Check sheet for the modelled part. Datum: model origin and axes. Units: mm. A direction names the side the tool comes from. Coordinates: 2 decimals unless noted, no trailing zeros. Loops run counter-clockwise (first coordinate to the right, second up) from the corner with the lowest first, then second, coordinate; pieces in that order, holes last. Notation, with made-up numbers: (51.5, 77) - (79.5, 77) arc R21 ccw to (79.5, 111) - close; hole circle Ø4 at (-29.75, 41.25). An arc over 180 degrees is marked (long way). Use a Markdown table: item, result. Add a question column.
1) Sectioned sample at A-A, the plane y = 6. Enter the section's corners in (x, z).
2) Go/stop test with flat-tipped pins: P1, Ø1.5, axis at x = 6, y = 3, coming from the +Z side; P2, Ø3.5, axis at y = 6, z = 0, coming from the -X side; P3, Ø3, axis at x = 4.5, y = 1, coming from the -Z side; P4, Ø2, axis at x = -1, z = -1.5, coming from the +Y side. Record where each tip stops, or that it passes through.
3) Draft check along Z on faces 4 (the cylindrical face through (-1.216, 0.021, 1.115)), 5 (the cylindrical face through (6.47, 8.93, 1.84)), 6 (the flat face through (5.4, 1.9, -2.6)). Enter one of: pulls with the +Z half, pulls with the -Z half, needs draft (parallel to the pull), parting line crosses it, or undercut.
4) Tool access check on faces 1 (the flat face through (7.741, 3, 0)), 2 (the flat face through (5.4, 1.9, 2.443)), 3 (the flat face through (2, 1.5, 0)). Record the directions out of +Z, -Z, +X, -X, +Y, -Y that give a thin tool (end or side, any length) a straight path to the whole face; none if there is none.
5) Sectioned sample at D-D, the plane x = 4. Enter the section's corners in (y, z).
6) Sectioned sample at C-C, the plane z = 0. Enter the section's corners in (x, y), then the cut area to 3 significant figures.
7) Sectioned sample at B-B, the plane x = 0. Enter the section's corners in (y, z).
8) Thickness scan on line 1 (Z direction, x = 6, y = 6); line 2 (Z direction, x = 0, y = 0.8); line 3 (X direction, y = 1.75, z = 0.45). Record the ranges inside material, lowest first.
from build123d import *

# Parameters (mm, degrees)
F0_R          = 3
F0_R_2        = 1.65
F1_DEPTH      = 1.5
F1_DEPTH_BACK = 1.5
F3_DEPTH      = 1.5
F3_DEPTH_BACK = 1.5
F4_W          = 2.5
F4_H          = 5.04355
F5_DEPTH      = 8
F6_R          = 2.05
F7_DEPTH      = 25
F8_R          = 2


with BuildPart() as f1:
    # F0 (on Front) → F1 (new body, two sides)
    with BuildSketch(Plane.XZ) as f1_sk:
        Circle(F0_R)
        Circle(F0_R_2, mode=Mode.SUBTRACT)
    extrude(amount=F1_DEPTH)
    extrude(f1_sk.sketch, amount=-F1_DEPTH_BACK)

    # F2 (on Front) → F3 (join, two sides)
    with BuildSketch(Plane.XZ) as f3_sk:
        with BuildLine():
            Line((7.740623, 2.443406), (1.740623, 2.443406))
            ThreePointArc((1.740623, 2.443406), (2.666633, 1.374433), (3, 0))
            ThreePointArc((3, 0), (2.59704, -1.501793), (1.496413, -2.600144))
            Line((1.496413, -2.600144), (7.740623, -2.600144))
            Line((7.740623, -2.600144), (7.740623, 2.443406))
        make_face()
    extrude(amount=F3_DEPTH)
    extrude(f3_sk.sketch, amount=-F3_DEPTH_BACK)

    # F4 (on face) → F5 (join)
    with BuildSketch(Plane(origin=(0, 1.5, 0), x_dir=(-1, 0, 0), z_dir=(0, 1, 0))):
        with Locations((-6.490623, -0.078369)):
            Rectangle(F4_W, F4_H)
    extrude(amount=F5_DEPTH)

    # F6 (on face) → F7 (cut)
    with BuildSketch(Plane(origin=(5.240623, 0, 0), x_dir=(0, -1, 0), z_dir=(-1, 0, 0))):
        with Locations((-6, 0)):
            Circle(F6_R)
    extrude(amount=-F7_DEPTH, mode=Mode.SUBTRACT)

    # F8
    f8_edges = [f1.edges().sort_by_distance(p)[0] for p in [
        (6.490623, 9.5, -2.600144),
        (6.490623, 9.5, 2.443406),
    ]]
    fillet(f8_edges, radius=F8_R)


solid = f1.part
Solved:
| question | item | result |
|---|---|---|
| 1 | outline | (5.24, -2.6) - (7.74, -2.6) - (7.74, -2.05) - (5.24, -2.05) - close; (5.24, 2.05) - (7.74, 2.05) - (7.74, 2.44) - (5.24, 2.44) - close |
| 2 | P1 | stops at z = 2.44 |
| 2 | P2 | passes through |
| 2 | P3 | stops at z = -2.6 |
| 2 | P4 | stops at y = 1.5 |
| 3 | face 4 | undercut |
| 3 | face 5 | pulls with the +Z half |
| 3 | face 6 | pulls with the -Z half |
| 4 | face 1 | +Z, -Z, +X, +Y, -Y |
| 4 | face 2 | +Z, +X, +Y, -Y |
| 4 | face 3 | +Z, -Z, -X, +Y |
| 5 | outline | (-1.5, -2.6) - (1.5, -2.6) - (1.5, 2.44) - (-1.5, 2.44) - close |
| 6 | outline | (-3, -1.5) - (-1.65, -1.5) - (-1.65, 1.5) - (-3, 1.5) - close; (1.65, -1.5) - (7.74, -1.5) - (7.74, 3.95) - (5.24, 3.95) - (5.24, 1.5) - (1.65, 1.5) - close; (5.24, 8.05) - (7.74, 8.05) - (7.74, 9.5) - (5.24, 9.5) - close |
| 6 | area | 32.1 mm2 |
| 7 | outline | (-1.5, -3) - (1.5, -3) - (1.5, -1.65) - (-1.5, -1.65) - close; (-1.5, 1.65) - (1.5, 1.65) - (1.5, 3) - (-1.5, 3) - close |
| 8 | line 1 | z = -2.6 to -2.05, 2.05 to 2.44 |
| 8 | line 2 | z = -3 to -1.65, 1.65 to 3 |
| 8 | line 3 | x = 5.24 to 7.74 |
